from build123d import *

# Parameters (mm, degrees)
SKETCH1_R           = 38
BOSS_EXTRUDE1_DEPTH = 24
SHELL1_T            = -3.5
SKETCH2_R           = 23.6
CUT_EXTRUDE1_DEPTH  = 3
SKETCH3_R           = 17.5
CUT_EXTRUDE2_DEPTH  = 0.5
BOSS_EXTRUDE2_START = -6
SKETCH4_R           = 44.5
SKETCH4_R_2         = 38
BOSS_EXTRUDE2_DEPTH = 6
SKETCH5_R           = 1.5
CUT_EXTRUDE3_DEPTH  = 6
CHAMFER1_SIZE       = 5


with BuildPart() as part:
    # Sketch1 → Boss-Extrude1 (new body)
    with BuildSketch(Plane.XY):
        Circle(SKETCH1_R)
    extrude(amount=BOSS_EXTRUDE1_DEPTH)

    # Shell1
    shell1_openings = [part.faces().sort_by_distance(p)[0] for p in [
        (0, 0, 24),
    ]]
    offset(amount=SHELL1_T, openings=shell1_openings, kind=Kind.INTERSECTION)

    # Sketch2 → Cut-Extrude1 (cut)
    with BuildSketch(Plane.XY.offset(3.5)):
        Circle(SKETCH2_R)
    extrude(amount=-CUT_EXTRUDE1_DEPTH, mode=Mode.SUBTRACT)

    # Sketch3 → Cut-Extrude2 (cut)
    with BuildSketch(Plane.XY.offset(0.5)):
        Circle(SKETCH3_R)
    extrude(amount=-CUT_EXTRUDE2_DEPTH, mode=Mode.SUBTRACT)

    # Sketch4 → Boss-Extrude2 (add)
    with BuildSketch(Plane.XY.offset(24).offset(BOSS_EXTRUDE2_START)):
        Circle(SKETCH4_R)
        Circle(SKETCH4_R_2, mode=Mode.SUBTRACT)
    extrude(amount=BOSS_EXTRUDE2_DEPTH)

    # Sketch5 → Cut-Extrude3 (cut)
    with BuildSketch(Plane.XY.offset(24)):
        with Locations((0, -41.5)):
            Circle(SKETCH5_R)
        with Locations((-41.5, 0)):
            Circle(SKETCH5_R)
        with Locations((0, 41.5)):
            Circle(SKETCH5_R)
        with Locations((41.5, 0)):
            Circle(SKETCH5_R)
    extrude(amount=-CUT_EXTRUDE3_DEPTH, mode=Mode.SUBTRACT)

    # Chamfer1
    chamfer1_edges = [part.edges().sort_by_distance(p)[0] for p in [
        (-34.5, 0, 24),
    ]]
    chamfer(chamfer1_edges, length=CHAMFER1_SIZE)

    # Chamfer2
    # the kernel refuses this chamfer: 5 mm, written as the material it adds along each edge
    with BuildSketch(Plane(origin=(0, 0, 18), x_dir=(1, 0, 0), z_dir=(0, -1, 0))) as chamfer2_piece_1_section:
        with BuildLine():
            Line((43.141421356, 0.141421356), (37.858578644, -5.141421356))
            Line((37.858578644, -5.141421356), (37.758578644, -5.141421356))
            ThreePointArc((37.758578644, -5.141421356), (37.9, -2.570710678), (37.9, 0))
            Line((37.9, 0), (38, 0.1))
            ThreePointArc((38, 0.1), (40.570710678, 0.1), (43.141421356, 0.241421356))
            Line((43.141421356, 0.241421356), (43.141421356, 0.141421356))
        make_face()
    chamfer2_piece_1 = revolve(axis=Axis((0, 0, 18), (0, 0, 1)), mode=Mode.PRIVATE)
    chamfer2_piece_1 = chamfer2_piece_1 - Plane(origin=(0, -41.5, 17.367076612), x_dir=(1, 0, 0), z_dir=(0, 0, 1)) * Cylinder(1.5, 173, mode=Mode.PRIVATE)
    chamfer2_piece_1 = chamfer2_piece_1 - Plane(origin=(41.5, 0, 17.367076612), x_dir=(1, 0, 0), z_dir=(0, 0, 1)) * Cylinder(1.5, 173, mode=Mode.PRIVATE)
    chamfer2_piece_1 = chamfer2_piece_1 - Plane(origin=(-41.5, 0, 17.367076612), x_dir=(1, 0, 0), z_dir=(0, 0, 1)) * Cylinder(1.5, 173, mode=Mode.PRIVATE)
    chamfer2_piece_1 = chamfer2_piece_1 - Plane(origin=(0, 41.5, 17.367076612), x_dir=(1, 0, 0), z_dir=(0, 0, 1)) * Cylinder(1.5, 173, mode=Mode.PRIVATE)
    add(chamfer2_piece_1)


solid = part.part
Here's how the part is built. I have some questions about the finished solid (model axes, mm). A direction names the side the tool comes from. Give positions to 0.01 mm unless a question says otherwise; leave off trailing zeros. Order: outer loops, then holes, each group sorted by start corner. A loop starts at its lowest first (then second) coordinate and runs counter-clockwise, first axis right, second up. Notation, with made-up numbers: (-19, -10.5) -> (0, -10.5) arc R20 ccw to (0, 5.5) -> close; hole circle Ø1 at (25.5, 28). An arc over 180 degrees is marked (long way). Use a Markdown table: item, result. Add a question column.
Item 1: Imagine slicing it at A-A on z = 21.5. Please give me the cut outline in (x, y), plus the area to 3 significant figures.
Item 2: Will these pins go through, and if not, where does the flat tip stop? pin 1 (1 mm diameter, centred on x = -35, z = 12.5, fed in from -Y); pin 2 (1 mm diameter, centred on y = 31.5, z = 10.5, fed in from -X); pin 3 (3.5 mm diameter, centred on x = 0, y = 41.5, fed in from -Z).
Item 3: For faces 5 (the face through (17.535, -33.713, 6.409)), 6 (the face through (-23.577, 1.038, 2.021)), 7 (the face through (0, 40, 21)), which set-ups out of +Z, -Z, +X, -X, +Y, -Y let a thin tool reach every point of the face, with its end or its side?
Item 4: I need wall thicknesses on line 1 (Y direction, x = 0, z = 1.7); line 2 (Y direction, x = 0, z = 0.1); line 3 (Y direction, x = 0, z = 19.5). Which ranges of each line are inside material? Lowest first, please.
Item 5: If we mould it in two halves opening along X, with no side actions, what happens to faces 1 (the face through (-32.798, 30.075, 20.958)), 2 (the face through (-18, 0, 0.5)), 3 (the face through (-0.2, 39.8, 24)), 4 (the face through (0, -40, 21))? For each: pulls with the +X half, pulls with the -X half, needs draft (parallel to the pull), parting line crosses it, or undercut.
Item 6: Imagine slicing it at B-B on z = 5.5. Please give me the cut outline in (x, y).
Data:
| question | item | result |
|---|---|---|
| 1 | outline | circle Ø89 at (0, 0); hole circle Ø3 at (-41.5, 0); hole circle Ø74 at (0, 0); hole circle Ø3 at (0, -41.5); hole circle Ø3 at (0, 41.5); hole circle Ø3 at (41.5, 0) |
| 1 | area | 1,890 mm² |
| 2 | pin 1 | stops at y = -15.93 |
| 2 | pin 2 | stops at x = -21.98 |
| 2 | pin 3 | stops at z = 14.75 |
| 3 | face 5 | -Z |
| 3 | face 6 | +Z |
| 3 | face 7 | +Z, -Z |
| 4 | line 1 | y = -38 to -23.6, 23.6 to 38 |
| 4 | line 2 | y = -38 to -17.5, 17.5 to 38 |
| 4 | line 3 | y = -44.5 to -43, -40 to -35, 35 to 40, 43 to 44.5 |
| 5 | face 1 | parting line crosses it |
| 5 | face 2 | undercut |
| 5 | face 3 | needs draft |
| 5 | face 4 | undercut |
| 6 | outline | circle Ø76 at (0, 0); hole circle Ø69 at (0, 0) |
